Part model, mm, in its own coordinate system. Face numbers are marked on the shaded views. Give positions to 0.01 mm unless a question says otherwise; leave off trailing zeros. Loops run counter-clockwise (first coordinate to the right, second up) from the corner with the lowest first, then second, coordinate; pieces in that order, holes last. Notation, with made-up numbers: M 9.5,-27 L 32.5,-27 A20 ccw 32.5,12 Z; hole C 29,29 d8. An arc over 180 degrees is marked long. Answer in a Markdown table with one row per item.
Autodesk Inventor part; units mm, degrees
ref_plane "YZ Plane" through (0, 0, 0) normal (1, 0, 0) x (0, 1, 0)
ref_plane "XZ Plane" through (0, 0, 0) normal (0, 1, 0) x (-1, 0, 0)
ref_plane "XY Plane" through (0, 0, 0) normal (0, 0, 1) x (1, 0, 0)
sketch "Sketch1" plane through (0, 0, 0) normal (0, 0, 1) x (1, 0, 0)
  line L0 (0, 0) -> (30.48, 0)
  line L1 (30.48, 0) -> (30.48, 16.002)
  line L2 (30.48, 16.002) -> (0, 16.002)
  line L3 (0, 16.002) -> (0, 0)
  dimension "d0" = 30.48
  dimension "d1" = 16.002
extrude "Extrusion1" add sketch "Sketch1" along normal blind 12.7
sketch "Sketch2" plane through (0, 0, 12.7) normal (0, 0, 1) x (1, 0, 0)
  line L0 (0, 0) -> (30.48, 0)
  line L1 (0, 16.002) -> (0, 0)
  point P0 (1.778, 8.001)
  point P1 (28.702, 14.224)
  point P2 (28.702, 1.778)
  dimension "d4" = 26.924
  dimension "d5" = 8.001
  dimension "d6" = 1.778
  dimension "d7" = 1.778
  dimension "d8" = 12.446
hole "Hole1" at (1.778, 8.001, 12.7) at (28.702, 14.224, 12.7) at (28.702, 1.778, 12.7) direction (0, 0, -1) diameter 2.54 end through all
sketch "Sketch3" plane through (30.48, 0, 0) normal (1, 0, 0) x (0, 0, -1)
  circle A0 centre (-7.62, 8.001) radius 0.381
  line L0 (-12.7, 0) -> (-12.7, 16.002)
  line L1 (0, 0) -> (-12.7, 0)
  dimension "d17" = 0.762
  dimension "d18" = 5.08
  dimension "d19" = 8.001
extrude "Extrusion2" add sketch "Sketch3" along normal blind 3.81
sketch "Sketch4" plane through (30.48, 0, 0) normal (1, 0, 0) x (0, 0, -1)
  line L0 (-4.8958, 4.826) -> (-3.9719, 6.4262)
  line L1 (-3.9719, 6.4262) -> (-2.1241, 6.4262)
  line L2 (-2.1241, 6.4262) -> (-1.2002, 4.826)
  line L3 (-1.2002, 4.826) -> (-2.1241, 3.2258)
  line L4 (-2.1241, 3.2258) -> (-3.9719, 3.2258)
  line L5 (-3.9719, 3.2258) -> (-4.8958, 4.826)
  line L6 (-3.9719, 3.2258) -> (-2.1241, 6.4262) construction
  line L7 (-2.1241, 3.2258) -> (-3.9719, 6.4262) construction
  line L8 (-12.7, 0) -> (-12.7, 16.002)
  line L9 (0, 0) -> (-12.7, 0)
  point P0 (-3.048, 4.826)
  point P1 (-3.048, 4.826)
  dimension "d22" = 120
  dimension "d23" = 9.652
  dimension "d24" = 4.826
  dimension "d25" = 3.2004
extrude "Extrusion3" add sketch "Sketch4" along normal blind 0.889
sketch "Sketch5" plane through (31.369, 0, 0) normal (1, 0, 0) x (0, 0, -1)
  line L0 (-3.9719, 3.2258) -> (-2.1241, 3.2258)
  line L1 (-1.2002, 4.826) -> (-2.1241, 6.4262)
  line L2 (-3.9719, 3.2258) -> (-2.1241, 6.4262)
  line L3 (-1.2002, 4.826) -> (-4.8958, 4.826)
  circle A0 centre (-3.048, 4.826) radius 0.8255
  point P0 (0, 0)
  dimension "d28" = 1.651
extrude "Extrusion4" add sketch "Sketch5" along normal blind 3.048 contours A0 L2 L3 | L3 L2 A0 | L2 L3 A0 | L2 A0 L3
sketch "Sketch6" plane through (34.417, 4.826, 3.048) normal (1, 0, 0) x (0, 0, -1)
  circle A0 centre (0, 0) radius 1.27
  circle A1 centre (0, 0) radius 0.8255
  point P0 (3.048, -4.826)
  dimension "d31" = 2.54
extrude "Extrusion5" add sketch "Sketch6" along normal blind 0.762 contours A0 | A1
properties part number "BTBody"
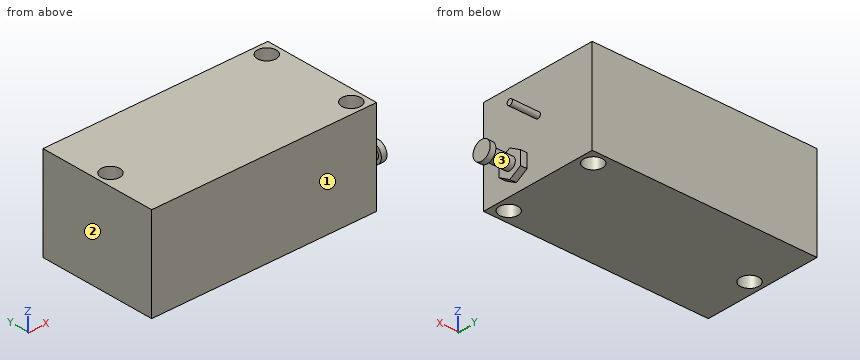
(1) Drill centre lines: line 1 along Y through (x, z) = (28, 7.25); line 2 along X through (y, z) = (9.5, 4.75); line 3 along X through (y, z) = (14.5, 11). Where is each one in solid material? Low to high.
Recorded:
| item | result |
|---|---|
| line 1 | y = 0 to 0.72, 2.84 to 13.17, 15.28 to 16 |
| line 2 | x = 0 to 30.48 |
| line 3 | x = 0 to 27.46, 29.94 to 30.48 |
(2) Saw through at C-C (z = 3.25). Write the cut outline in (x, y).
Recorded:
| item | result |
|---|---|
| outline | M 0,0 L 30.48,0 L 30.48,3.23 L 31.37,3.23 L 31.37,4.03 L 34.42,4.03 L 34.42,3.57 L 35.18,3.57 L 35.18,6.08 L 34.42,6.08 L 34.42,5.63 L 31.37,5.63 L 31.37,6.43 L 30.48,6.43 L 30.48,16 L 0,16 Z; hole C 1.78,8 d2.54; hole C 28.7,1.78 d2.54; hole C 28.7,14.22 d2.54 |
(3) Saw through at B-B (y = 14.5). Write the cut outline in (x, z).
Recorded:
| item | result |
|---|---|
| outline | M 0,0 L 27.46,0 L 27.46,12.7 L 0,12.7 Z; M 29.94,0 L 30.48,0 L 30.48,12.7 L 29.94,12.7 Z |
(4) Saw through at D-D (z = 9.5). Write the cut outline in (x, y), plus the area to 3 significant figures.
Recorded:
| item | result |
|---|---|
| outline | M 0,0 L 30.48,0 L 30.48,16 L 0,16 Z; hole C 1.78,8 d2.54; hole C 28.7,1.78 d2.54; hole C 28.7,14.22 d2.54 |
| area | 473 mm^2 |
(5) Pull direction X, two halves, no side cores. Call the marked faces 1, 2 and 3: +X half, -X half, draft (parallel to the pull), parting line (faces both ways), or undercut.
Recorded:
| item | result |
|---|---|
| face 1 | draft |
| face 2 | -X half |
| face 3 | undercut |
(6) Pin check, flat tips, straight feed: pin 1 Ø2 at (y, z) = (12, 2) entering from -X; pin 2 Ø1.5 at (x, y) = (1.778, 8.001) entering from -Z; pin 3 Ø4 at (y, z) = (10.5, 11) entering from +X. Stop position of each tip, or through.
Recorded:
| item | result |
|---|---|
| pin 1 | stops at x = 0 |
| pin 2 | passes through |
| pin 3 | stops at x = 30.48 |
(7) Saw through at A-A (z = 7.62). Write the cut outline in (x, y), plus the area to 3 significant figures.
Recorded:
| item | result |
|---|---|
| outline | M 0,0 L 30.48,0 L 30.48,7.62 L 34.29,7.62 L 34.29,8.38 L 30.48,8.38 L 30.48,16 L 0,16 Z; hole C 1.78,8 d2.54; hole C 28.7,1.78 d2.54; hole C 28.7,14.22 d2.54 |
| area | 475 mm^2 |
